```python
from build123d import *

# Parameters (mm, degrees)
F1_W     = 68.9904686213
F1_H     = 3.5
F2_DEPTH = 3
F3_R     = 1.74999


# Not quite as in the source:
# - a fillet or chamfer is up to 0.001 mm smaller than in the source, because OpenCascade refuses the exact size


with BuildPart() as f2:
    # F1 (on Top) → F2 (new body)
    with BuildSketch(Plane.XY):
        with BuildLine():
            Line((0, 10.5), (0, 0))
            Line((0, 0), (89.0564994759, 0))
            ThreePointArc((89.0564994759, 0), (79.609277662, 2.8667059749), (73.3482214035, 10.5))
            Line((73.3482214035, 10.5), (59.6541650593, 10.5))
            Line((59.6541650593, 10.5), (0, 10.5))
        make_face()
        with Locations((37.9952343106, 5.25)):
            Rectangle(F1_W, F1_H, mode=Mode.SUBTRACT)
        with BuildLine():
            ThreePointArc((73.3482214035, 10.5), (79.609277662, 2.8667059749), (89.0564994759, 0))
            ThreePointArc((89.0564994759, 0), (101.0773147561, 4.9791847198), (106.0564994759, 17))
            ThreePointArc((106.0564994759, 17), (105.1713324233, 22.414070472), (102.6080101728, 27.2643342614))
            Line((102.6080101728, 27.2643342614), (95.6259965732, 24.5393439959))
            ThreePointArc((95.6259965732, 24.5393439959), (98.158558885, 21.1415594301), (99.0564994759, 17))
            ThreePointArc((99.0564994759, 17), (88.5076755448, 7.0150717432), (79.1167410173, 18.0959935155))
            Line((79.1167410173, 18.0959935155), (72.1347274177, 15.37100325))
            ThreePointArc((72.1347274177, 15.37100325), (72.5606905825, 12.8904636571), (73.3482214035, 10.5))
        make_face()
    extrude(amount=F2_DEPTH)

    # F3 (radius 1.75 in the source; OpenCascade refuses exactly that, so slightly less here)
    f3_edges = [f2.edges().sort_by_distance(p)[0] for p in [
        (3.5, 7, 1.5),
        (3.5, 3.5, 1.5),
        (0, 10.5, 1.5),
        (0, 0, 1.5),
        (72.490469, 7, 1.5),
        (72.490469, 3.5, 1.5),
    ]]
    fillet(f3_edges, radius=F3_R)


solid = f2.part
```
Verification items for the finished model (mm, model axes). A direction names the side the tool comes from. Coordinates: 2 decimals unless noted, no trailing zeros. Order: outer loops, then holes, each group sorted by start corner. A loop starts at its lowest first (then second) coordinate and runs counter-clockwise, first axis right, second up. Notation, with made-up numbers: (73, 29.25) -> (125, 29.25) arc R15 cw to (125, 48.25) -> close; hole circle Ø9 at (36.25, 82.5). An arc over 180 degrees is marked (long way). Put each result on its own line as item: value. Start each with the question number.
1) Cross-section at C-C (y = 13). Enter the section's corners in (x, z).
2) Cross-section at D-D (x = 84). Enter the section's corners in (y, z), plus the area to 3 significant figures.
3) Tool access check on faces 4 (the flat face through (38, 3.5, 1)), 5 (the flat face through (0, 5, 1)). Record the directions out of +Z, -Z, +X, -X, +Y, -Y that give a thin tool (end or side, any length) a straight path to the whole face; none if there is none.
4) Material ranges on L1, parallel to Y at x = 7, z = 2.2; L2, parallel to X at y = 8.75, z = 0.6; L3, parallel to X at y = 7.75, z = 0.8, recorded low to high.
5) Go/stop test with a flat-tipped pin: pin 1 (1.5 mm diameter, centred on y = 12.5, z = 2, fed in from -X). Record where the tip stops, or that it passes through.
6) Release check for a two-part mould opening along Y. For faces 1 (the cylindrical face through (72.552, 12.925, 1.479)), 2 (the flat face through (61, 10, 3)), 3 (the cylindrical face through (0.499, 0.526, 1.521)) record: pulls with the +Y half, pulls with the -Y half, needs draft (parallel to the pull), parting line crosses it, or undercut.
7) Cross-section at A-A (x = 54). Enter the section's corners in (y, z).
Geometry check:
1. outline: (72.53, 0) -> (79.89, 0) -> (79.89, 3) -> (72.53, 3) -> close; (98.22, 0) -> (105.58, 0) -> (105.58, 3) -> (98.22, 3) -> close
2. outline: (0, 0) -> (8.37, 0) -> (8.37, 3) -> (0, 3) -> close
2. area: 25.1 mm^2
3. face 4: +Z, -Z
3. face 5: +Z, -Z, -X, +Y, -Y
4. L1: y = 0 to 3.5, 7 to 10.5
4. L2: x = 0 to 83.41, 94.71 to 103.92
4. L3: x = 0 to 85.26, 92.86 to 103.32
5. pin 1: stops at x = 72.48
6. face 1: undercut
6. face 2: needs draft
6. face 3: pulls with the -Y half
7. outline: (0, 0) -> (3.5, 0) -> (3.5, 3) -> (0, 3) -> close; (7, 0) -> (10.5, 0) -> (10.5, 3) -> (7, 3) -> close
